Here's how the part is built. I have some questions about the finished solid (model axes, mm). Face numbers are marked on the shaded views. A direction names the side the tool comes from. Coordinates: 2 decimals unless noted, no trailing zeros. Write each loop counter-clockwise with the first axis right and the second up, starting at its lowest first coordinate (ties: lowest second). Pieces come first, ordered by that corner, then holes.
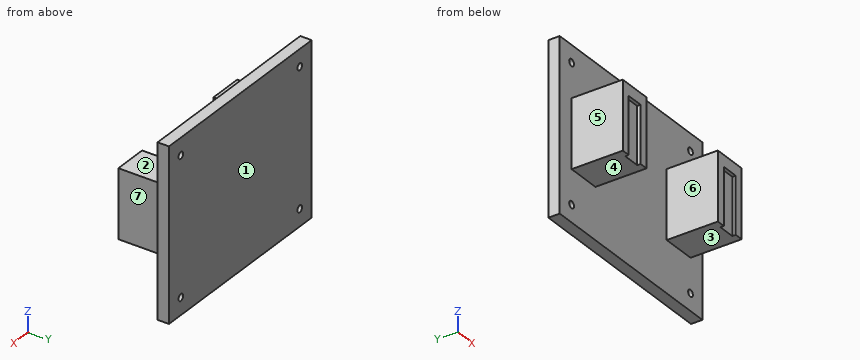
```python
from build123d import *

# Parameters (mm, degrees)
IZIM1_W                     = 180
IZIM1_H                     = 150
Y_KSEKLIK_EKSTR_ZYON1_DEPTH = 10
IZIM2_R                     = 3
KES_EKSTR_ZYON1_DEPTH       = 35
IZIM3_W                     = 30
IZIM3_H                     = 60
Y_KSEKLIK_EKSTR_ZYON2_DEPTH = 45
IZIM5_W                     = 15
IZIM5_H                     = 3
KES_EKSTR_ZYON2_DEPTH       = 50
IZIM7_W                     = 15
IZIM7_H                     = 3
KES_EKSTR_ZYON3_DEPTH       = 50


with BuildPart() as part:
    # Çizim1 → Yükseklik-Ekstrüzyon1 (new body)
    with BuildSketch(Plane(origin=(0, 0, 0), x_dir=(1, 0, 0), z_dir=(0, 1, 0))):
        Rectangle(IZIM1_W, IZIM1_H)
    extrude(amount=Y_KSEKLIK_EKSTR_ZYON1_DEPTH)

    # Çizim2 → Kes-Ekstrüzyon1 (cut)
    with BuildSketch(Plane(origin=(0, 10, 0), x_dir=(1, 0, 0), z_dir=(0, 1, 0))):
        with Locations(Location((-75, 60, 0), (0, 0, 270))):
            Circle(IZIM2_R)
        with Locations(Location((-75, -60, 0), (0, 0, 270))):
            Circle(IZIM2_R)
        with Locations(Location((75, -60, 0), (0, 0, 270))):
            Circle(IZIM2_R)
        with Locations(Location((75, 60, 0), (0, 0, 270))):
            Circle(IZIM2_R)
    extrude(amount=-KES_EKSTR_ZYON1_DEPTH, mode=Mode.SUBTRACT)

    # Çizim3 → Yükseklik-Ekstrüzyon2 (add)
    with BuildSketch(Plane.XZ):
        with Locations((-60, 0)):
            Rectangle(IZIM3_W, IZIM3_H)
        with Locations((60, 0)):
            Rectangle(IZIM3_W, IZIM3_H)
    extrude(amount=Y_KSEKLIK_EKSTR_ZYON2_DEPTH)

    # Çizim5 → Kes-Ekstrüzyon2 (cut)
    with BuildSketch(Plane(origin=(0, 0, -30), x_dir=(-1, 0, 0), z_dir=(0, 0, -1))):
        with Locations((60, -43.5)):
            Rectangle(IZIM5_W, IZIM5_H)
    extrude(amount=-KES_EKSTR_ZYON2_DEPTH, mode=Mode.SUBTRACT)

    # Çizim7 → Kes-Ekstrüzyon3 (cut)
    with BuildSketch(Plane(origin=(0, 0, -30), x_dir=(-1, 0, 0), z_dir=(0, 0, -1))):
        with Locations((-60, -43.5)):
            Rectangle(IZIM7_W, IZIM7_H)
    extrude(amount=-KES_EKSTR_ZYON3_DEPTH, mode=Mode.SUBTRACT)


solid = part.part
```
1) Imagine slicing it at A-A on z = 60. Please give me the cut outline in (x, y), then the cut area to 3 significant figures.
Values follow:
outline: (-90, 0) - (-78, 0) - (-78, 10) - (-90, 10) - close; (-72, 0) - (72, 0) - (72, 10) - (-72, 10) - close; (78, 0) - (90, 0) - (90, 10) - (78, 10) - close
area: 1,680 mm2
2) Imagine slicing it at D-D on z = 5.5. Please give me the cut outline in (x, y), then the cut area to 3 significant figures.
Values follow:
outline: (-90, 0) - (-75, 0) - (-75, -45) - (-67.5, -45) - (-67.5, -42) - (-52.5, -42) - (-52.5, -45) - (-45, -45) - (-45, 0) - (45, 0) - (45, -45) - (52.5, -45) - (52.5, -42) - (67.5, -42) - (67.5, -45) - (75, -45) - (75, 0) - (90, 0) - (90, 10) - (-90, 10) - close
area: 4,410 mm2
3) On a 3-axis mill with a long thin cutter (end or side, diameter ignored), from which of +Z, -Z, +X, -X, +Y, -Y can I reach the whole of each face in a straight line? I mean the marked faces 1, 2 and 3. Say none if no direction works.
Values follow:
face 1: +Z, -Z, +X, -X, +Y
face 2: +Z, +X, -X, -Y
face 3: -Z, +X, -X, -Y
4) Imagine slicing it at B-B on y = -27.5. Please give me the cut outline in (x, z), then the cut area to 3 significant figures.
Values follow:
outline: (-75, -30) - (-45, -30) - (-45, 30) - (-75, 30) - close; (45, -30) - (75, -30) - (75, 30) - (45, 30) - close
area: 3,600 mm2
5) Imagine slicing it at C-C on x = -18. Please give me the cut outline in (y, z).
Values follow:
outline: (0, -75) - (10, -75) - (10, 75) - (0, 75) - close
6) We'd pull the mould along X, two halves only. Please class the marked faces 4, 5, 6 and 7: pulls with the +X half, pulls with the -X half, needs draft (parallel to the pull), parting line crosses it, or undercut.
Values follow:
face 4: needs draft
face 5: pulls with the -X half
face 6: undercut
face 7: pulls with the +X half
7) I need wall thicknesses on probe 1 along X at (y, z) = (4, 60); probe 2 along X at (y, z) = (-27, -24.5); probe 3 along Z at (x, y) = (49, -36). Which ranges of each line are inside material? Lowest first, please.
Values follow:
probe 1: x = -90 to -78, -72 to 72, 78 to 90
probe 2: x = -75 to -45, 45 to 75
probe 3: z = -30 to 30
8) Will these pins go through, and if not, where does the flat tip stop? pin 1 (4 mm diameter, centred on x = 56, z = -45, fed in from -Y); pin 2 (2.5 mm diameter, centred on y = -43, z = -2, fed in from -X); pin 3 (3.5 mm diameter, centred on x = -75, z = -60, fed in from +Y); pin 4 (3 mm diameter, centred on y = -4.5, z = -21.5, fed in from +X).
Values follow:
pin 1: stops at y = 0
pin 2: stops at x = -75
pin 3: passes through
pin 4: stops at x = 75
